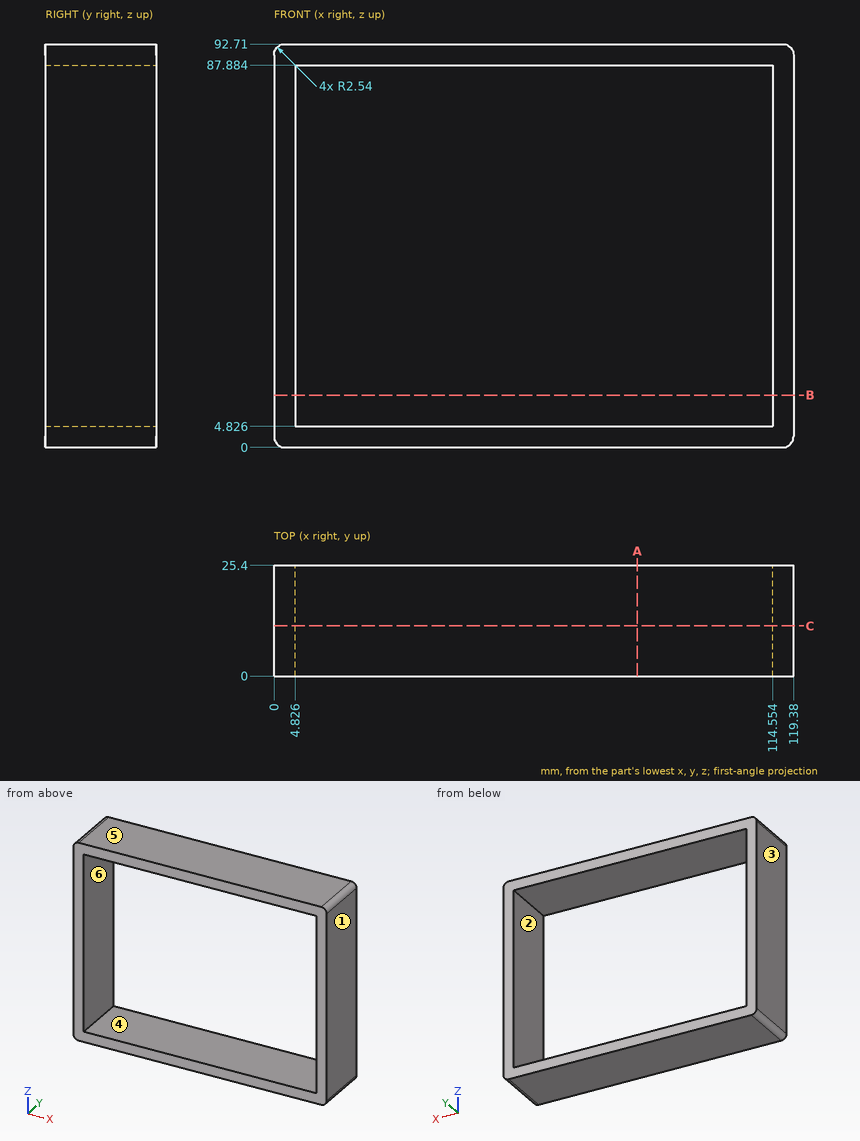
Study the drawing (mm; zero at the part's minimum x, y, z) and answer. A direction names the side the tool comes from. Round coordinates to 2 decimals unless told otherwise and drop trailing zeros. Write each loop counter-clockwise with the first axis right and the second up, starting at its lowest first coordinate (ties: lowest second). Pieces come first, ordered by that corner, then holes.
1) A cutting plane is placed at C-C (y = 11.5). Give the vertices of the cut face in (x, z), plus the area to 3 significant figures.
2) A cutting plane is placed at A-A (x = 83.5). Give the vertices of the cut face in (y, z), plus the area to 3 significant figures.
3) A cutting plane is placed at B-B (z = 12). Give the vertices of the cut face in (x, y), plus the area to 3 significant figures.
4) The mould has two halves that part along Z. Classify the marked faces 3, 4, 5 and 6: pulls with the +Z half, pulls with the -Z half, needs draft (parallel to the pull), parting line crosses it, or undercut.
5) Given pin 1 Ø10 at (x, z) = (45, 14) entering from -Y, flat-ended and moving along its own axis, determine where the tip first touches the part or whether it passes through.
6) A tool of negligible diameter and unlimited length cuts with its end or side. For the marked faces 1 and 2, from which of +Z, -Z, +X, -X, +Y, -Y can it reach the whole face along a straight path? Write none if from no direction.
7) Straight lines are drawn through the part: line 1 (Z direction, x = 49, y = 7); line 2 (X direction, y = 8, z = 72). For each, find the intervals that lie inside material, in ascending order.
Completed:
1. outline: (0, 2.54) arc R2.54 ccw to (2.54, 0) - (116.84, 0) arc R2.54 ccw to (119.38, 2.54) - (119.38, 90.17) arc R2.54 ccw to (116.84, 92.71) - (2.54, 92.71) arc R2.54 ccw to (0, 90.17) - close; hole (4.83, 4.83) - (114.55, 4.83) - (114.55, 87.88) - (4.83, 87.88) - close
1. area: 1,950 mm2
2. outline: (0, 0) - (25.4, 0) - (25.4, 4.83) - (0, 4.83) - close; (0, 87.88) - (25.4, 87.88) - (25.4, 92.71) - (0, 92.71) - close
2. area: 245 mm2
3. outline: (0, 0) - (4.83, 0) - (4.83, 25.4) - (0, 25.4) - close; (114.55, 0) - (119.38, 0) - (119.38, 25.4) - (114.55, 25.4) - close
3. area: 245 mm2
4. face 3: needs draft
4. face 4: undercut
4. face 5: pulls with the +Z half
4. face 6: undercut
5. pin 1: passes through
6. face 1: +Z, -Z, +X, +Y, -Y
6. face 2: +Y, -Y
7. line 1: z = 0 to 4.83, 87.88 to 92.71
7. line 2: x = 0 to 4.83, 114.55 to 119.38
